Verification items for the finished model (mm, model axes). Round coordinates to 2 decimals unless told otherwise and drop trailing zeros. Write each loop counter-clockwise with the first axis right and the second up, starting at its lowest first coordinate (ties: lowest second). Pieces come first, ordered by that corner, then holes. Notation, with made-up numbers: (74, -26.5) - (96, -26.5) arc R23 cw to (96, -14.5) - close; hole circle Ø11 at (-22.75, 22.25). An arc over 180 degrees is marked (long way). Answer as a JSON object with one key per item and string values.
```python
from build123d import *

# Parameters (mm, degrees)
SKETCH1_R           = 4
BOSS_EXTRUDE1_DEPTH = 2.5


with BuildPart() as part:
    # Sketch1 → Boss-Extrude1 (new, symmetric)
    with BuildSketch(Plane.YZ):
        with BuildLine():
            Line((-16, 0), (16, 0))
            Line((16, 0), (8.779015578, 31.982141641))
            ThreePointArc((8.779015578, 31.982141641), (0, 39), (-8.779015578, 31.982141641))
            Line((-8.779015578, 31.982141641), (-16, 0))
        make_face()
        with Locations(Location((0, 30, 0), (0, 0, 270))):
            Circle(SKETCH1_R, mode=Mode.SUBTRACT)
    extrude(amount=BOSS_EXTRUDE1_DEPTH, both=True)


solid = part.part
```
1. Go/stop test with flat-tipped pins: pin 1 (3 mm diameter, centred on x = 1.5, y = 4.5, fed in from +Z); pin 2 (1 mm diameter, centred on x = 1.5, z = 20.5, fed in from +Y); pin 3 (1.5 mm diameter, centred on x = -1.5, z = 6, fed in from +Y). Record where each tip stops, or that it passes through.
Completed:
{"pin 1": "stops at z = 38.49", "pin 2": "stops at y = 11.48", "pin 3": "stops at y = 14.81"}
2. Cross-section at B-B (x = -1.85). Record the boundary of the cut face in (y, z), plus the area to 3 significant figures.
Completed:
{"outline": "(-16, 0) - (16, 0) - (8.78, 31.98) arc R9 ccw to (-8.78, 31.98) - close; hole circle Ø8 at (0, 30)", "area": "834 mm^2"}
3. Cross-section at D-D (y = 5). Record the boundary of the cut face in (x, z), plus the area to 3 significant figures.
Completed:
{"outline": "(-2.5, 0) - (2.5, 0) - (2.5, 37.48) - (-2.5, 37.48) - close", "area": "187 mm^2"}
4. Mould release check, pull along Y, two halves, no side actions. Record for faces 1 (the face through (0, 0, 39)), 2 (the face through (0, -2.4, 33.2)), 3 (the face through (0.04, 12.44, 15.77)): released by +Y, released by -Y, zero draft, split by the parting line, or undercut.
Completed:
{"face 1": "split by the parting line", "face 2": "undercut", "face 3": "released by +Y"}
5. Cross-section at C-C (z = 30). Record the boundary of the cut face in (x, y), plus the area to 3 significant figures.
Completed:
{"outline": "(-2.5, -9.23) - (2.5, -9.23) - (2.5, -4) - (-2.5, -4) - close; (-2.5, 4) - (2.5, 4) - (2.5, 9.23) - (-2.5, 9.23) - close", "area": "52.3 mm^2"}
6. Cross-section at A-A (y = 0). Record the boundary of the cut face in (x, z).
Completed:
{"outline": "(-2.5, 0) - (2.5, 0) - (2.5, 26) - (-2.5, 26) - close; (-2.5, 34) - (2.5, 34) - (2.5, 39) - (-2.5, 39) - close"}
7. Material ranges on probe 1 along Z at (x, y) = (0.9, 1); probe 2 along Y at (x, z) = (1.1, 30); probe 3 along Z at (x, y) = (1.45, 1.5), recorded low to high. Write a range as from..to.
Completed:
{"probe 1": "z = 0..26.13, 33.87..38.94", "probe 2": "y = -9.23..-4, 4..9.23", "probe 3": "z = 0..26.29, 33.71..38.87"}
